Autodesk Inventor part; units mm, degrees
ref_plane "YZ Plane" through (0, 0, 0) normal (1, 0, 0) x (0, 1, 0)
ref_plane "XZ Plane" through (0, 0, 0) normal (0, 1, 0) x (-1, 0, 0)
ref_plane "XY Plane" through (0, 0, 0) normal (0, 0, 1) x (1, 0, 0)
sketch "Sketch1" plane through (0, 0, 0) normal (0, 1, 0) x (-1, 0, 0)
  circle A0 centre (0, 0) radius 13.5
  circle A1 centre (0, 0) radius 11.5
  line L0 (0, 0) -> (13.099, 3.2659)
  line L1 (0, 0) -> (13.099, -3.2659)
  line L2 (0, 0) -> (13.5, 0)
  circle A2 centre (0, 0) radius 10 construction
  line L3 (0, 0) -> (10.5058, 4.6775)
  line L4 (0, 0) -> (10.5058, -4.6775)
  arc A3 (9.703, 2.4192) -> (9.1355, 4.0674) centre (0, 0) ccw
  arc A4 (9.1355, -4.0674) -> (9.703, -2.4192) centre (0, 0) ccw
  arc A5 (9.1355, 4.0674) -> (9.6593, 6.2409) centre (6.4382, 5.8673) ccw
  arc A6 (9.1462, -6.9711) -> (9.1355, -4.0674) centre (7.2505, -5.5263) ccw
  circle A7 centre (11.3253, 3.4202) radius 0.5578
  circle A8 centre (11.3253, -3.4202) radius 0.5578
  point P0 (11.1584, 2.7821)
  point P1 (11.1584, -2.7821)
  dimension "d0" = 27
  dimension "d1" = 23
  dimension "d2" = 14
  dimension "d3" = 14
  dimension "d4" = 20
  dimension "d5" = 10
  dimension "d6" = 10
extrude "Extrusion1" add sketch "Sketch1" along normal blind 1.5 contours L0 A1 A7 A8 L1 A0 | L0 A3 L3 A1 A7 | A1 A8 L4 A4 L1 | A7 A1 | A1 A7 | A8 A1 | A1 A8 | A5 A1 L3 | L4 A1 A6
properties part number "20_Cube_Insert_Beamsplittercube_Retainring_25mm"
Design review of the part built by this model. Coordinates are the model's own, in mm. A direction names the side the tool comes from. Coordinates: 2 decimals unless noted, no trailing zeros. Order: outer loops, then holes, each group sorted by start corner. A loop starts at its lowest first (then second) coordinate and runs counter-clockwise, first axis right, second up. Notation, with made-up numbers: (29.5, 80.5) - (33.5, 80.5) arc R21 ccw to (33.5, 108.5) - close; hole circle Ø8 at (68.25, 78). An arc over 180 degrees is marked (long way). Answer in a Markdown table with one row per item.
(1) Consider section C-C on y = 1.25. State the section outline as (x, z) points, plus the area to 3 significant figures.
Checked values:
| item | result |
|---|---|
| outline | (-13.1, -3.27) arc R13.5 ccw (long way) to (-13.1, 3.27) - (-9.7, 2.42) arc R10 cw to (-9.14, 4.07) arc R3.24 cw to (-9.66, 6.24) arc R11.5 cw (long way) to (-9.15, -6.97) arc R2.38 cw to (-9.14, -4.07) arc R10 cw to (-9.7, -2.42) - close |
| area | 153 mm^2 |
(2) Consider section A-A on x = 0. State the section outline as (y, z) points.
Checked values:
| item | result |
|---|---|
| outline | (0, -13.5) - (1.5, -13.5) - (1.5, -11.5) - (0, -11.5) - close; (0, 11.5) - (1.5, 11.5) - (1.5, 13.5) - (0, 13.5) - close |
(3) The part is to be moulded in two halves that separate along Z. For faces 4 (the cylindrical face through (-9.594, 0.74, 5.123)), 5 (the cylindrical face through (13.49, 0.74, -0.55)), 6 (the flat face through (-10, 1.5, -3)), 7 (the flat face through (-11.377, 0.74, 2.837)), say which applies: released by +Z, released by -Z, zero draft, split by the parting line, or undercut.
Checked values:
| item | result |
|---|---|
| face 4 | undercut |
| face 5 | split by the parting line |
| face 6 | zero draft |
| face 7 | undercut |
(4) Consider section B-B on z = 10.5. State the section outline as (x, y) points.
Checked values:
| item | result |
|---|---|
| outline | (-8.49, 0) - (-4.69, 0) - (-4.69, 1.5) - (-8.49, 1.5) - close; (4.69, 0) - (8.49, 0) - (8.49, 1.5) - (4.69, 1.5) - close |
(5) Wall thickness on line 1 along Z through (x, y) = (0, 1.05); line 2 along Z through (x, y) = (-5.5, 0.75); line 3 along X through (y, z) = (0.9, -10): over which ranges is each line inside the solid? List them lowest first. Write a range as from..to.
Checked values:
| item | result |
|---|---|
| line 1 | -13.5..-11.5, 11.5..13.5 |
| line 2 | -12.33..-10.1, 10.1..12.33 |
| line 3 | -9.07..-5.68, 5.68..9.07 |
(6) Consider section D-D on z = 0. State the section outline as (x, y) points, plus the area to 3 significant figures.
Checked values:
| item | result |
|---|---|
| outline | (11.5, 0) - (13.5, 0) - (13.5, 1.5) - (11.5, 1.5) - close |
| area | 3.00 mm^2 |
(7) For faces 1 (the flat face through (-10, 0, -3)), 2 (the cylindrical face through (-9.634, 0.74, -5.496)), 3 (the flat face through (-11.377, 0.74, -2.837)), list the 3-axis set-ups (+Z, -Z, +X, -X, +Y, -Y) from which the entire face can be reached by the end or side of a thin tool; tool diameter is ignored.
Checked values:
| item | result |
|---|---|
| face 1 | +Z, -Z, +X, -X, -Y |
| face 2 | +Y, -Y |
| face 3 | -X, +Y, -Y |
